Part model, mm, in its own coordinate system. A direction names the side the tool comes from. Coordinates: 2 decimals unless noted, no trailing zeros. Write each loop counter-clockwise with the first axis right and the second up, starting at its lowest first coordinate (ties: lowest second). Pieces come first, ordered by that corner, then holes. Notation, with made-up numbers: (22, -38) -> (73, -38) arc R11 ccw to (73, -27) -> close; hole circle Ø9 at (36.5, 14). An arc over 180 degrees is marked (long way). Write item = value, one per line. Start each with the question number.
Q1. Tool access for faces 5 (the flat face through (-15, -53, -1)), 6 (the flat face through (0, -25, 0)): list every direction of +Z, -Z, +X, -X, +Y, -Y with a clear straight run to the whole face (end or side of a thin tool).
Q2. Pin check, flat tips, straight feed: P1, Ø7, axis at x = -25, y = -7.48, coming from the +Z side; P2, Ø0.9, axis at y = -47, z = -1, coming from the -X side; P3, Ø0.8, axis at x = -13.5, z = -1.5, coming from the -Y side; P4, Ø0.5, axis at x = 13.5, z = -1.5, coming from the -Y side. Stop position of each tip, or through.
Q3. Band-saw the part on A-A, the plane x = 0. List the corners of the cut face in (y, z).
Q4. Band-saw the part on D-D, the plane z = -1.45. Give the number of separate pieces and of enclosed holes in the cut face, plus the area to 3 significant figures.
Q5. Pull direction X, two halves, no side cores. Call faces 1 (the flat face through (-15, -44, -1)), 2 (the flat face through (0, -25, -3)), 3 (the flat face through (15, -44, -1)), 4 (the flat face through (14.854, -59.692, -1.479)): released by +X, released by -X, zero draft, split by the parting line, or undercut.
Q6. Probe line 1 (X direction, y = -42, z = -0.7); line 2 (Y direction, x = -12.5, z = -1.6); line 3 (X direction, y = -6, z = -1.15). List the from-to ranges inside material, lowest first.
Q7. Band-saw the part on C-C, the plane x = -25. List the corners of the cut face in (y, z), plus the area to 3 significant figures.
Q8. Band-saw the part on B-B, the plane y = -44. List the corners of the cut face in (x, z).
from build123d import *

# Parameters (mm, degrees)
SKETCH1_R            = 2.6
SKETCH1_R_2          = 1.25
BASE_FLANGE1_DEPTH   = 3
FILLET1_R            = 5
FILLET2_R            = 10
CUT_EXTRUDE1_REACH   = 74.507
SKETCH3_W            = 3
SKETCH3_H            = 6.5
FILLET3_R            = 1
FILLET3_OF_MIRROR1_R = 1
FILLET4_R            = 5


# Sheet-metal steps are written as plain solids
with BuildPart() as part:
    # Sketch1 → Base-Flange1 (new body)
    with BuildSketch(Plane.XY):
        Polygon((-31, -0.476720525), (31, -0.476720525), (31, -35.476720525), (19, -35.476720525), (19, -54.752062511), (10, -65.476720525), (-10, -65.476720525), (-19, -54.752062511), (-19, -35.476720525), (-31, -35.476720525), align=None)
        with Locations((25, -7.476720525)):
            Circle(SKETCH1_R, mode=Mode.SUBTRACT)
        with Locations((-25, -7.476720525)):
            Circle(SKETCH1_R, mode=Mode.SUBTRACT)
        with Locations((-12.5, -27.476720525)):
            Circle(SKETCH1_R_2, mode=Mode.SUBTRACT)
        with Locations((12.5, -27.476720525)):
            Circle(SKETCH1_R_2, mode=Mode.SUBTRACT)
        with Locations((12.5, -7.476720525)):
            Circle(SKETCH1_R_2, mode=Mode.SUBTRACT)
        with Locations((-12.5, -7.476720525)):
            Circle(SKETCH1_R_2, mode=Mode.SUBTRACT)
        with BuildLine():
            Line((-2.6, -50.076720525), (-2.6, -44.876720525))
            ThreePointArc((-2.6, -44.876720525), (0, -42.276720525), (2.6, -44.876720525))
            Line((2.6, -44.876720525), (2.6, -50.076720525))
            ThreePointArc((2.6, -50.076720525), (0, -52.676720525), (-2.6, -50.076720525))
        make_face(mode=Mode.SUBTRACT)
    extrude(amount=-BASE_FLANGE1_DEPTH)

    # Fillet1
    fillet1_edges = [part.edges().sort_by_distance(p)[0] for p in [
        (-31, -0.476720525, -1.5),
        (31, -0.476720525, -1.5),
    ]]
    fillet(fillet1_edges, radius=FILLET1_R)

    # Fillet2
    fillet2_edges = [part.edges().sort_by_distance(p)[0] for p in [
        (31, -35.476720525, -1.5),
        (19, -54.752062511, -1.5),
        (10, -65.476720525, -1.5),
        (-10, -65.476720525, -1.5),
        (-19, -54.752062511, -1.5),
        (-31, -35.476720525, -1.5),
    ]]
    fillet(fillet2_edges, radius=FILLET2_R)

    # Sketch3 → Cut-Extrude1 (cut, up to next)
    with BuildSketch(Plane.XY, mode=Mode.PRIVATE) as cut_extrude1_sk1:
        with Locations((13.5, -44.326720525)):
            Rectangle(SKETCH3_W, SKETCH3_H)
    cut_extrude1_tool1 = extrude(cut_extrude1_sk1.sketch, amount=-CUT_EXTRUDE1_REACH, mode=Mode.PRIVATE) & part.part
    # Sketch3 → Cut-Extrude1 (cut, up to next)
    with BuildSketch(Plane.XY, mode=Mode.PRIVATE) as cut_extrude1_sk2:
        with Locations((13.5, -53.326720525)):
            Rectangle(SKETCH3_W, SKETCH3_H)
    cut_extrude1_tool2 = extrude(cut_extrude1_sk2.sketch, amount=-CUT_EXTRUDE1_REACH, mode=Mode.PRIVATE) & part.part
    cut_extrude1_1 = cut_extrude1_tool1.solids().sort_by_distance((13.5, -44.326721, 0))[0]
    add(cut_extrude1_1, mode=Mode.SUBTRACT)
    cut_extrude1_2 = cut_extrude1_tool2.solids().sort_by_distance((13.5, -53.326721, 0))[0]
    add(cut_extrude1_2, mode=Mode.SUBTRACT)
    cut_extrude1 = cut_extrude1_1 + cut_extrude1_2  # Cut-Extrude1 as one shape, for the pattern or mirror that repeats it

    # Fillet3
    fillet3_edges = [part.edges().sort_by_distance(p)[0] for p in [
        (12, -47.576720525, -1.5),
        (12, -41.076720525, -1.5),
        (15, -41.076720525, -1.5),
        (15, -47.576720525, -1.5),
        (12, -56.576720525, -1.5),
        (12, -50.076720525, -1.5),
        (15, -50.076720525, -1.5),
        (15, -56.576720525, -1.5),
    ]]
    fillet(fillet3_edges, radius=FILLET3_R)

    # Mirror1: Cut-Extrude1 across plane
    add(cut_extrude1.mirror(Plane(origin=(0, 0, 0), x_dir=(0, 0, 1), z_dir=(1, 0, 0))), mode=Mode.SUBTRACT)

    # Fillet3 of Mirror1
    fillet3_of_mirror1_edges = [part.edges().sort_by_distance(p)[0] for p in [
        (-12, -47.576720525, -1.5),
        (-12, -41.076720525, -1.5),
        (-15, -41.076720525, -1.5),
        (-15, -47.576720525, -1.5),
        (-12, -56.576720525, -1.5),
        (-12, -50.076720525, -1.5),
        (-15, -50.076720525, -1.5),
        (-15, -56.576720525, -1.5),
    ]]
    fillet(fillet3_of_mirror1_edges, radius=FILLET3_OF_MIRROR1_R)

    # Fillet4
    fillet4_edges = [part.edges().sort_by_distance(p)[0] for p in [
        (19, -35.476720525, -1.5),
        (-19, -35.476720525, -1.5),
    ]]
    fillet(fillet4_edges, radius=FILLET4_R)


solid = part.part
Ans:
q1.face_5 = +Z, -Z
q1.face_6 = +Z, +X, -X, +Y, -Y
q2.P1 = 0
q2.P2 = -19
q2.P3 = -61.78
q2.P4 = -61.6
q3.outline = (-65.48, -3) -> (-52.68, -3) -> (-52.68, 0) -> (-65.48, 0) -> close; (-42.28, -3) -> (-0.48, -3) -> (-0.48, 0) -> (-42.28, 0) -> close
q4.separate_pieces = 1
q4.enclosed_holes = 11
q4.area = 2,970 mm2
q5.face_1 = undercut
q5.face_2 = zero draft
q5.face_3 = undercut
q5.face_4 = released by +X
q6.line_1 = -19 to -15, -12 to 12, 15 to 19
q6.line_2 = -62.45 to -56.44, -50.21 to -47.44, -41.21 to -28.73, -26.23 to -8.73, -6.23 to -0.48
q6.line_3 = -31 to -27.14, -22.86 to 22.86, 27.14 to 31
q7.outline = (-34.64, -3) -> (-10.08, -3) -> (-10.08, 0) -> (-34.64, 0) -> close; (-4.88, -3) -> (-0.48, -3) -> (-0.48, 0) -> (-4.88, 0) -> close
q7.area = 86.9 mm2
q8.outline = (-19, -3) -> (-15, -3) -> (-15, 0) -> (-19, 0) -> close; (-12, -3) -> (-2.45, -3) -> (-2.45, 0) -> (-12, 0) -> close; (2.45, -3) -> (12, -3) -> (12, 0) -> (2.45, 0) -> close; (15, -3) -> (19, -3) -> (19, 0) -> (15, 0) -> close
